from build123d import *

# Parameters (mm, degrees)
F3_W     = 31.95
F3_H     = 31.86
F3_R     = 2.05
F3_R_2   = 3.955
F4_DEPTH = 1.9304
F1_W     = 31.95
F1_H     = 31.86
F1_R     = 2.05
F1_R_2   = 3.955
F5_DEPTH = 1.9304
F5_TAPER = -3


with BuildPart() as f4:
    # F3 (on offset) → F4 (new body)
    with BuildSketch(Plane.YZ.offset(16.002)):
        Rectangle(F3_W, F3_H)
        with Locations((0, -7.62)):
            Circle(F3_R, mode=Mode.SUBTRACT)
        with Locations((-7.62, 0)):
            Circle(F3_R, mode=Mode.SUBTRACT)
        Circle(F3_R_2, mode=Mode.SUBTRACT)
        with Locations((7.62, 0)):
            Circle(F3_R, mode=Mode.SUBTRACT)
        with Locations((0, 7.62)):
            Circle(F3_R, mode=Mode.SUBTRACT)
    extrude(amount=F4_DEPTH)

    # F1 (on offset) → F5 (join)
    with BuildSketch(Plane.XY.offset(-16.002)):
        Rectangle(F1_W, F1_H)
        with Locations((0, -7.62)):
            Circle(F1_R, mode=Mode.SUBTRACT)
        with Locations((-7.62, 0)):
            Circle(F1_R, mode=Mode.SUBTRACT)
        Circle(F1_R_2, mode=Mode.SUBTRACT)
        with Locations((7.62, 0)):
            Circle(F1_R, mode=Mode.SUBTRACT)
        with Locations((0, 7.62)):
            Circle(F1_R, mode=Mode.SUBTRACT)
    extrude(amount=F5_DEPTH, taper=F5_TAPER)


solid = f4.part
Geometry check sheet. Reference: the model listing, model coordinates, mm. A direction names the side the tool comes from. Coordinates: 2 decimals unless noted, no trailing zeros. Order: outer loops, then holes, each group sorted by start corner. A loop starts at its lowest first (then second) coordinate and runs counter-clockwise, first axis right, second up. Notation, with made-up numbers: (70.25, 39.5) -> (116.25, 39.5) arc R18 ccw to (116.25, 69.5) -> close; hole circle Ø6 at (12.25, 16.5). An arc over 180 degrees is marked (long way). Use a Markdown table: item, result. Add a question column.
1. Material ranges on L1, parallel to Z at x = 17.2, y = 0 (3 decimals); L2, parallel to Z at x = 17.4, y = 7.62; L3, parallel to X at y = 6.5, z = 14, recorded low to high.
2. Cross-section at A-A (z = 7.62). Enter the section's corners in (x, y) (3 decimals).
3. Go/stop test with flat-tipped pins: pin 1 Ø1 at (x, z) = (17, -7.5) entering from -Y (3 decimals); pin 2 Ø1.5 at (x, y) = (8, 9.5) entering from +Z; pin 3 Ø3.5 at (y, z) = (0, 7.62) entering from -X; pin 4 Ø12.5 at (y, z) = (0, 0) entering from -X. Record where each tip stops, or that it passes through.
4. Mould release check, pull along Y, two halves, no side actions. Record for faces 4 (the face through (17, 15.975, 0)), 5 (the face through (17.932, 3, 4)), 6 (the face through (-3.09, 2.37, -14.81)): pulls with the +Y half, pulls with the -Y half, needs draft (parallel to the pull), parting line crosses it, or undercut.
5. Cross-section at B-B (z = -1.5). Enter the section's corners in (x, y) (3 decimals).
6. Cross-section at C-C (x = 0). Give the number of separate pieces and of enclosed holes in the cut face, and give its area (3 significant figures).
7. Set-up check for faces 1 (the face through (-0.26, 5.64, -15.02)), 2 (the face through (-4, 4, -14.072)), 3 (the face through (17, 0, -15.93)): record each of +Z, -Z, +X, -X, +Y, -Y from which the full face is reachable in a straight line by a thin tool's end or side.
Filled sheet:
| question | item | result |
|---|---|---|
| 1 | L1 | -15.93 to -9.67, -5.57 to -3.955, 3.955 to 5.57, 9.67 to 15.93 |
| 1 | L2 | -15.93 to -2.05, 2.05 to 15.93 |
| 1 | L3 | 16 to 17.93 |
| 2 | outline | (16.002, -15.975) -> (17.932, -15.975) -> (17.932, -2.05) -> (16.002, -2.05) -> close; (16.002, 2.05) -> (17.932, 2.05) -> (17.932, 15.975) -> (16.002, 15.975) -> close |
| 3 | pin 1 | y = -15.975 |
| 3 | pin 2 | z = -14.07 |
| 3 | pin 3 | through |
| 3 | pin 4 | x = 16 |
| 4 | face 4 | pulls with the +Y half |
| 4 | face 5 | needs draft |
| 4 | face 6 | undercut |
| 5 | outline | (16.002, -15.975) -> (17.932, -15.975) -> (17.932, -9.017) -> (16.002, -9.017) -> close; (16.002, -6.223) -> (17.932, -6.223) -> (17.932, -3.66) -> (16.002, -3.66) -> close; (16.002, 3.66) -> (17.932, 3.66) -> (17.932, 6.223) -> (16.002, 6.223) -> close; (16.002, 9.017) -> (17.932, 9.017) -> (17.932, 15.975) -> (16.002, 15.975) -> close |
| 6 | separate pieces | 4 |
| 6 | enclosed holes | 0 |
| 6 | area | 31.2 mm2 |
| 7 | face 1 | -Z |
| 7 | face 2 | +Z, -X, +Y, -Y |
| 7 | face 3 | -Z, +X, +Y, -Y |
